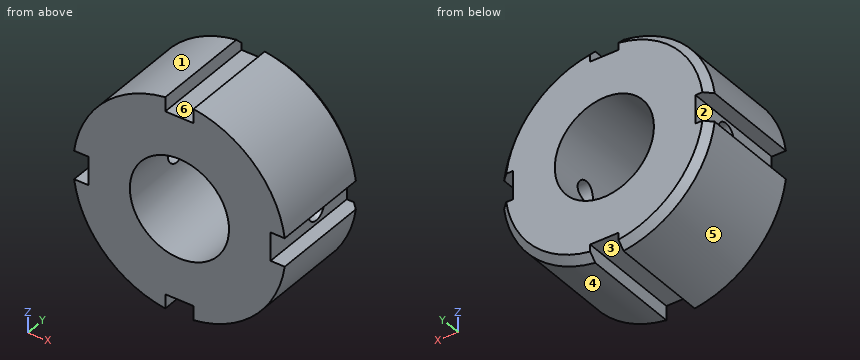
from build123d import *

# Parameters (mm, degrees)
SKETCH1_R               = 15
BOSS_EXTRUDE1_DEPTH     = 7.5
CUT_EXTRUDE1_DEPTH      = 8.5
CUT_EXTRUDE1_DEPTH_BACK = 8.5
CHAMFER1_SIZE           = 1
M16_TAPPED_HOLE1_D      = 14
M16_TAPPED_HOLE1_DEPTH  = 15
SKETCH5_R               = 1.5
CUT_EXTRUDE2_DEPTH      = 3
CUT_EXTRUDE2_DEPTH_BACK = 28.732137495


with BuildPart() as part:
    # Sketch1 → Boss-Extrude1 (new body, symmetric)
    with BuildSketch(Plane(origin=(0, 0, 0), x_dir=(1, 0, 0), z_dir=(0, 1, 0))):
        Circle(SKETCH1_R)
    extrude(amount=BOSS_EXTRUDE1_DEPTH, both=True)

    # Sketch2 → Cut-Extrude1 (cut, two sides)
    with BuildSketch(Plane(origin=(0, 0, 0), x_dir=(1, 0, 0), z_dir=(0, 1, 0))) as cut_extrude1_sk:
        with BuildLine():
            Line((-2, 14.866068747), (-2, 12.866068747))
            Line((-2, 12.866068747), (2, 12.866068747))
            Line((2, 12.866068747), (2, 14.866068747))
            ThreePointArc((2, 14.866068747), (0, 15), (-2, 14.866068747))
        make_face()
        with BuildLine():
            Line((14.866068747, 2), (12.866068747, 2))
            Line((12.866068747, 2), (12.866068747, -2))
            Line((12.866068747, -2), (14.866068747, -2))
            ThreePointArc((14.866068747, -2), (15, 0), (14.866068747, 2))
        make_face()
        with BuildLine():
            Line((2, -14.866068747), (2, -12.866068747))
            Line((2, -12.866068747), (-2, -12.866068747))
            Line((-2, -12.866068747), (-2, -14.866068747))
            ThreePointArc((-2, -14.866068747), (0, -15), (2, -14.866068747))
        make_face()
        with BuildLine():
            Line((-14.866068747, -2), (-12.866068747, -2))
            Line((-12.866068747, -2), (-12.866068747, 2))
            Line((-12.866068747, 2), (-14.866068747, 2))
            ThreePointArc((-14.866068747, 2), (-15, 0), (-14.866068747, -2))
        make_face()
    extrude(amount=CUT_EXTRUDE1_DEPTH, mode=Mode.SUBTRACT)
    extrude(cut_extrude1_sk.sketch, amount=-CUT_EXTRUDE1_DEPTH_BACK, mode=Mode.SUBTRACT)

    # Chamfer1
    chamfer1_edges = [part.edges().sort_by_distance(p)[0] for p in [
        (10.606601718, 7.5, -10.606601718),
        (-10.606601718, 7.5, -10.606601718),
        (-10.606601718, 7.5, 10.606601718),
        (10.606601718, 7.5, 10.606601718),
    ]]
    chamfer(chamfer1_edges, length=CHAMFER1_SIZE)

    # M16 Tapped Hole1
    with Locations(Plane(origin=(0, 7.5, 0), x_dir=(1, 0, 0), z_dir=(0, 1, 0))):
        with Locations((0, 0)):
            Hole(M16_TAPPED_HOLE1_D / 2, depth=M16_TAPPED_HOLE1_DEPTH)

    # Sketch5 → Cut-Extrude2 (cut, two sides)
    with BuildSketch(Plane(origin=(12.866068747, 0, 0), x_dir=(0, 0, -1), z_dir=(1, 0, 0))) as cut_extrude2_sk:
        with Locations((0, 1.5)):
            Circle(SKETCH5_R)
    extrude(amount=CUT_EXTRUDE2_DEPTH, mode=Mode.SUBTRACT)
    extrude(cut_extrude2_sk.sketch, amount=-CUT_EXTRUDE2_DEPTH_BACK, mode=Mode.SUBTRACT)


solid = part.part
Model file for the job. Use its own axes, mm. Face numbers are marked on the shaded views. A direction names the side the tool comes from. Give positions to 0.01 mm unless a question says otherwise; leave off trailing zeros. Loops run counter-clockwise (first coordinate to the right, second up) from the corner with the lowest first, then second, coordinate; pieces in that order, holes last. Notation, with made-up numbers: (52, 27.5) -> (76, 27.5) arc R22 cw to (76, 50.5) -> close; hole circle Ø11 at (70.5, 75.5). An arc over 180 degrees is marked (long way). Use a Markdown table: item, result. Add a question column.
(1) Slice it at D-D on y = -1. List the corners of the cut face in (x, z), and give its area (3 significant figures).
(2) Slice it at C-C on z = 0. List the corners of the cut face in (x, y), and give its area (3 significant figures).
(3) Slice it at B-B on x = 0. List the corners of the cut face in (y, z).
(4) Slice it at A-A on y = 1.5. List the corners of the cut face in (x, z), and give its area (3 significant figures).
(5) Drop flat-ended pins along their axis: pin 1 Ø2 at (y, z) = (-1, 14) entering from +X; pin 2 Ø3 at (y, z) = (3.5, 0) entering from -X; pin 3 Ø4.5 at (x, y) = (0.5, 0) entering from -Z; pin 4 Ø1.5 at (x, z) = (-2, 5.5) entering from +Y. Give the stop position or say it passes through.
(6) Wall check: line 1 along Y through (x, z) = (11, 0); line 2 along X through (y, z) = (-2.5, -13.5); line 3 along X through (y, z) = (6.5, 4.25). Give the ranges that are in metal, low to high.
(7) Tool access for the marked faces 1 and 2: list every direction of +Z, -Z, +X, -X, +Y, -Y with a clear straight run to the whole face (end or side of a thin tool).
(8) Mould opens along X. For the marked faces 3, 4, 5 and 6 say: +X half, -X half, draft (parallel to the pull), parting line (faces both ways), or undercut.
Filled sheet:
| question | item | result |
|---|---|---|
| 1 | outline | (-14.87, -2) arc R15 ccw to (-2, -14.87) -> (-2, -12.87) -> (2, -12.87) -> (2, -14.87) arc R15 ccw to (14.87, -2) -> (12.87, -2) -> (12.87, 2) -> (14.87, 2) arc R15 ccw to (2, 14.87) -> (2, 12.87) -> (-2, 12.87) -> (-2, 14.87) arc R15 ccw to (-14.87, 2) -> (-12.87, 2) -> (-12.87, -2) -> close; hole circle Ø14 at (0, 0) |
| 1 | area | 519 mm2 |
| 2 | outline | (-12.87, -7.5) -> (-7, -7.5) -> (-7, 0) -> (-12.87, 0) -> close; (-12.87, 3) -> (-7, 3) -> (-7, 7.5) -> (-12.87, 7.5) -> close; (7, -7.5) -> (12.87, -7.5) -> (12.87, 0) -> (7, 0) -> close; (7, 3) -> (12.87, 3) -> (12.87, 7.5) -> (7, 7.5) -> close |
| 2 | area | 141 mm2 |
| 3 | outline | (-7.5, -12.87) -> (7.5, -12.87) -> (7.5, -7) -> (-7.5, -7) -> close; (-7.5, 7) -> (7.5, 7) -> (7.5, 12.87) -> (-7.5, 12.87) -> close |
| 4 | outline | (-14.87, -2) arc R15 ccw to (-2, -14.87) -> (-2, -12.87) -> (2, -12.87) -> (2, -14.87) arc R15 ccw to (14.87, -2) -> (12.87, -2) -> (12.87, -1.5) -> (6.84, -1.5) arc R7 cw to (-6.84, -1.5) -> (-12.87, -1.5) -> (-12.87, -2) -> close; (-14.87, 2) -> (-12.87, 2) -> (-12.87, 1.5) -> (-6.84, 1.5) arc R7 cw to (6.84, 1.5) -> (12.87, 1.5) -> (12.87, 2) -> (14.87, 2) arc R15 ccw to (2, 14.87) -> (2, 12.87) -> (-2, 12.87) -> (-2, 14.87) arc R15 ccw to start |
| 4 | area | 484 mm2 |
| 5 | pin 1 | x = 7.48 |
| 5 | pin 2 | x = -12.87 |
| 5 | pin 3 | z = -14.87 |
| 5 | pin 4 | through |
| 6 | line 1 | -7.5 to 0, 3 to 7.5 |
| 6 | line 2 | -6.54 to -2, 2 to 6.54 |
| 6 | line 3 | -14.39 to -5.56, 5.56 to 14.39 |
| 7 | face 1 | +Z, -X, +Y, -Y |
| 7 | face 2 | -X, +Y, -Y |
| 8 | face 3 | undercut |
| 8 | face 4 | +X half |
| 8 | face 5 | -X half |
| 8 | face 6 | undercut |
